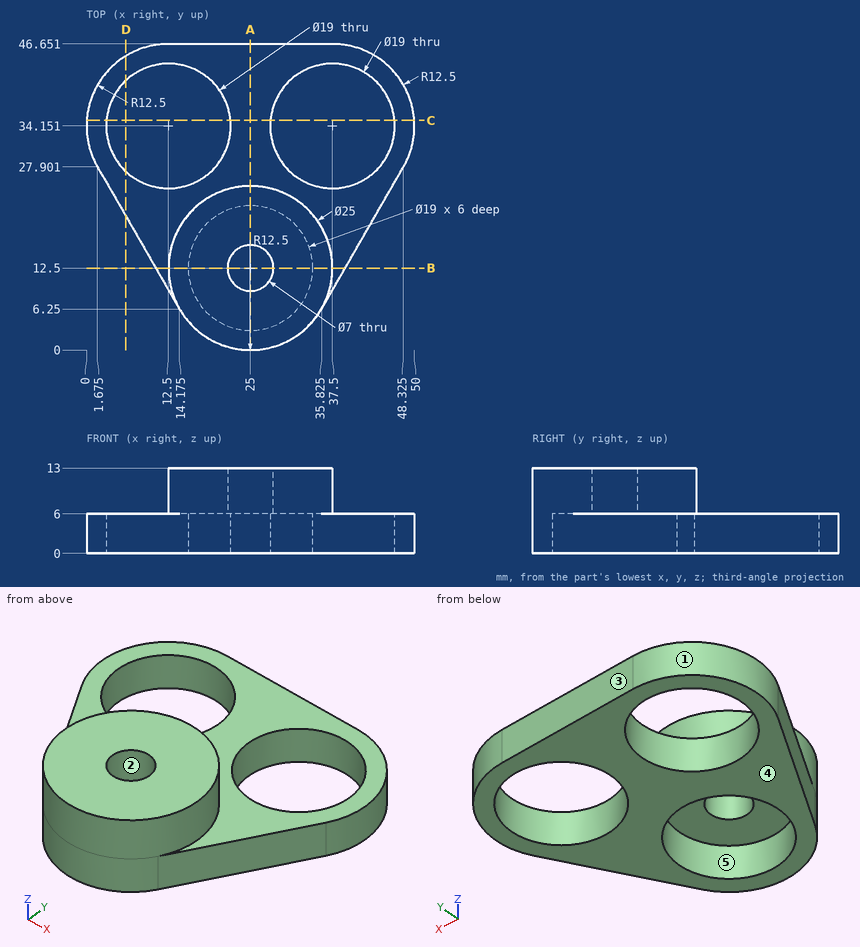
Verification items for this drawing (mm, ordinates from the low corner). A direction names the side the tool comes from. Coordinates: 2 decimals unless noted, no trailing zeros. Loops run counter-clockwise (first coordinate to the right, second up) from the corner with the lowest first, then second, coordinate; pieces in that order, holes last. Notation, with made-up numbers: (54, 7.25) - (93, 7.25) arc R15 ccw to (93, 23.25) - close; hole circle Ø7 at (67, 62). An arc over 180 degrees is marked (long way). One line per item, written item: value. Start each with the question number.
(1) Cross-section at A-A on x = 25. Enter the section's corners in (y, z).
(2) Depth check by flat-ended pin: P1, Ø24.5, axis at x = 25, y = 12.5, coming from the +Z side; P2, Ø5, axis at x = 28, z = 4.5, coming from the -Y side; P3, Ø4, axis at x = 9.5, z = 11.5, coming from the +Y side; P4, Ø1, axis at y = 14.5, z = 3.5, coming from the -X side. Enter the tip coordinate at first touch or a pass-through.
(3) Cross-section at B-B on y = 12.5. Enter the section's corners in (x, z).
(4) Cross-section at C-C on y = 35. Enter the section's corners in (x, z).
(5) Cross-section at D-D on x = 6. Enter the section's corners in (y, z).
(6) Tool access check on the marked faces 4 and 5. Record the directions out of +Z, -Z, +X, -X, +Y, -Y that give a thin tool (end or side, any length) a straight path to the whole face; none if there is none.
(7) Material ranges on line 1 (Y direction, x = 25, z = 11.75); line 2 (Z direction, x = 20.5, y = 20); line 3 (X direction, y = 15, z = 11.25), recorded low to high. Write a range as [from, to].
(8) Mould release check, pull along Y, two halves, no side actions. Record for the marked faces 1, 2 and 3: released by +Y, released by -Y, zero draft, split by the parting line, or undercut.
Results below:
1. outline: (0, 0) - (3, 0) - (3, 6) - (9, 6) - (9, 13) - (0, 13) - close; (16, 6) - (22, 6) - (22, 0) - (46.65, 0) - (46.65, 6) - (25, 6) - (25, 13) - (16, 13) - close
2. P1: stops at z = 13
2. P2: stops at y = 0.01
2. P3: passes through
2. P4: stops at x = 9.12
3. outline: (10.57, 0) - (15.5, 0) - (15.5, 6) - (21.5, 6) - (21.5, 13) - (12.5, 13) - (12.5, 6) - (10.57, 6) - close; (28.5, 6) - (34.5, 6) - (34.5, 0) - (39.43, 0) - (39.43, 6) - (37.5, 6) - (37.5, 13) - (28.5, 13) - close
4. outline: (0.03, 0) - (3.04, 0) - (3.04, 6) - (0.03, 6) - close; (21.96, 0) - (28.04, 0) - (28.04, 6) - (21.96, 6) - close; (46.96, 0) - (49.97, 0) - (49.97, 6) - (46.96, 6) - close
5. outline: (20.41, 0) - (27.22, 0) - (27.22, 6) - (20.41, 6) - close; (41.08, 0) - (44.83, 0) - (44.83, 6) - (41.08, 6) - close
6. face 4: -Z, +X, -X, +Y, -Y
6. face 5: -Z
7. line 1: y = [0, 9], [16, 25]
7. line 2: z = [6, 13]
7. line 3: x = [12.75, 22.55], [27.45, 37.25]
8. face 1: split by the parting line
8. face 2: undercut
8. face 3: released by +Y
